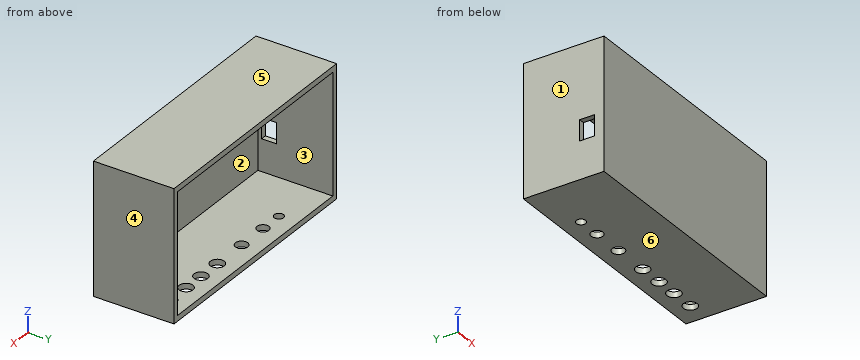
```python
from build123d import *

# Parameters (mm, degrees)
SKETCH5_W           = 130
SKETCH5_H           = 70
BOSS_EXTRUDE3_DEPTH = 43
SKETCH6_W           = 124
SKETCH6_H           = 64
CUT_EXTRUDE3_DEPTH  = 40
SKETCH8_R           = 3.7
CUT_EXTRUDE7_DEPTH  = 40
SKETCH9_R           = 3.3
SKETCH9_R_2         = 3.2
SKETCH9_R_3         = 2.5
CUT_EXTRUDE8_DEPTH  = 40
SKETCH10_W          = 11
SKETCH10_H          = 8
CUT_EXTRUDE9_DEPTH  = 40


with BuildPart() as part:
    # Sketch5 → Boss-Extrude3 (new body)
    with BuildSketch(Plane(origin=(0, 0, 0), x_dir=(1, 0, 0), z_dir=(0, 1, 0))):
        with Locations((65, -35)):
            Rectangle(SKETCH5_W, SKETCH5_H)
    extrude(amount=BOSS_EXTRUDE3_DEPTH)

    # Sketch6 → Cut-Extrude3 (cut)
    with BuildSketch(Plane(origin=(0, 43, 0), x_dir=(1, 0, 0), z_dir=(0, 1, 0))):
        with Locations((65, -35)):
            Rectangle(SKETCH6_W, SKETCH6_H)
    extrude(amount=-CUT_EXTRUDE3_DEPTH, mode=Mode.SUBTRACT)

    # Sketch8 → Cut-Extrude7 (cut)
    with BuildSketch(Plane(origin=(0, 0, 0), x_dir=(-1, 0, 0), z_dir=(0, 0, -1))):
        with Locations((-105, 32.75)):
            Circle(SKETCH8_R)
        with Locations((-93.081395349, 32.75)):
            Circle(SKETCH8_R)
        with Locations((-80, 32.75)):
            Circle(SKETCH8_R)
        with Locations((-118.081395349, 32.75)):
            Circle(SKETCH8_R)
    extrude(amount=-CUT_EXTRUDE7_DEPTH, mode=Mode.SUBTRACT)

    # Sketch9 → Cut-Extrude8 (cut)
    with BuildSketch(Plane(origin=(0, 0, 0), x_dir=(-1, 0, 0), z_dir=(0, 0, -1))):
        with Locations((-60.600049653, 32.75)):
            Circle(SKETCH9_R)
        with Locations((-43.4660788, 32.75)):
            Circle(SKETCH9_R_2)
        with Locations((-30.78166501, 32.75)):
            Circle(SKETCH9_R_3)
    extrude(amount=-CUT_EXTRUDE8_DEPTH, mode=Mode.SUBTRACT)

    # Sketch10 → Cut-Extrude9 (cut)
    with BuildSketch(Plane.ZY):
        with Locations((25.5, 9)):
            Rectangle(SKETCH10_W, SKETCH10_H)
    extrude(amount=-CUT_EXTRUDE9_DEPTH, mode=Mode.SUBTRACT)


solid = part.part
```
For this review, take the finished solid that the model builds, in its own axes (mm). Face numbers are marked on the shaded views. A direction names the side the tool comes from. Coordinates: 2 decimals unless noted, no trailing zeros. Loops run counter-clockwise (first coordinate to the right, second up) from the corner with the lowest first, then second, coordinate; pieces in that order, holes last.
1. Add section C-C, the plane y = 8.5. Give the boundary of the cut face in (x, z), then the cut area to 3 significant figures.
2. Add section B-B, the plane x = 105. Give the boundary of the cut face in (y, z), then the cut area to 3 significant figures.
3. For the marked faces 1 and 2, list the 3-axis set-ups (+Z, -Z, +X, -X, +Y, -Y) from which the entire face can be reached by the end or side of a thin tool; tool diameter is ignored.
4. Add section D-D, the plane y = 32.75. Count the separate pieces of the cut face and the enclosed holes in it, then the cut area to 3 significant figures.
5. Mouldability with a two-part tool opening along Z and no side actions: class the marked faces 3, 4, 5 and 6 as +Z half, -Z half, draft (parallel to the pull), parting line (faces both ways), or undercut.
6. For line 1 (X direction, y = 7.5, z = 35.5); line 2 (Z direction, x = 37, y = 20.5); line 3 (Y direction, x = 105, z = 1.45), list the stretches that pass through material, from the lowest coordinate up.
7. Add section A-A, the plane z = 60. Give the boundary of the cut face in (x, y), then the cut area to 3 significant figures.
8. Insertion check: P1, Ø12, axis at x = 18.5, z = 48.5, coming from the +Y side. The pin has a flat end and moves straight along its axis. Give the tip position at first contact, or say it passes through.
Result:
1. outline: (0, 0) - (130, 0) - (130, 70) - (0, 70) - (0, 31) - (3, 31) - (3, 67) - (127, 67) - (127, 3) - (3, 3) - (3, 20) - (0, 20) - close
1. area: 1,130 mm2
2. outline: (0, 0) - (29.05, 0) - (29.05, 3) - (3, 3) - (3, 67) - (43, 67) - (43, 70) - (0, 70) - close; (36.45, 0) - (43, 0) - (43, 3) - (36.45, 3) - close
2. area: 428 mm2
3. face 1: +Z, -Z, -X, +Y, -Y
3. face 2: +Y
4. separate pieces: 7
4. enclosed holes: 0
4. area: 1,020 mm2
5. face 3: undercut
5. face 4: draft
5. face 5: +Z half
5. face 6: -Z half
6. line 1: x = 0 to 3, 127 to 130
6. line 2: z = 0 to 3, 67 to 70
6. line 3: y = 0 to 29.05, 36.45 to 43
7. outline: (0, 0) - (130, 0) - (130, 43) - (127, 43) - (127, 3) - (3, 3) - (3, 43) - (0, 43) - close
7. area: 630 mm2
8. P1: stops at y = 3
